For this review, take the finished solid that the model builds, in its own axes (mm). Give positions to 0.01 mm unless a question says otherwise; leave off trailing zeros. Write each loop counter-clockwise with the first axis right and the second up, starting at its lowest first coordinate (ties: lowest second). Pieces come first, ordered by that corner, then holes. Notation, with made-up numbers: M 29.25,64 L 69.25,64 A9 cw 69.25,77 Z; hole C -37,43.5 d3. An arc over 180 degrees is marked long. Answer as a JSON object with one key per item and string values. Group by question number.
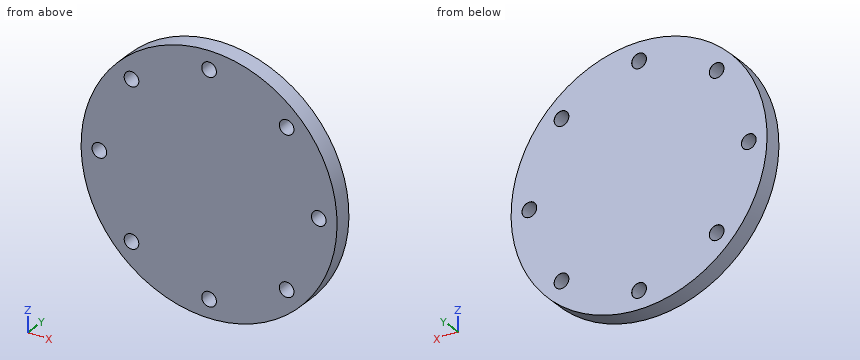
```python
from build123d import *

# Parameters (mm, degrees)
SKETCH_1_W                   = 70
SKETCH_1_H                   = 10
HOLE_WIZARD_M8_1_D           = 8
HOLE_WIZARD_M8_1_CSINK_D     = 8.05
HOLE_WIZARD_M8_1_CSINK_ANGLE = 100
PATTERN_CIRCULAR_2_COUNT     = 8


with BuildPart() as part:
    # Sketch 1 → Revolve 1 (revolve)
    with BuildSketch(Plane.XY, mode=Mode.PRIVATE) as revolve_1_sk:
        with Locations((-35, 5)):
            Rectangle(SKETCH_1_W, SKETCH_1_H)
    revolve(revolve_1_sk.sketch.rotate(Axis((0, 76.619497233, 0), (0, -1, 0)), 270), axis=Axis((0, 76.619497233, 0), (0, -1, 0)))

    # Hole Wizard M8 _1 (through all)
    with Locations(Plane(origin=(0, 10, 0), x_dir=(1, 0, 0), z_dir=(0, 1, 0))):
        with Locations((-60, 0)):
            hole_wizard_m8_1 = CounterSinkHole(HOLE_WIZARD_M8_1_D / 2, HOLE_WIZARD_M8_1_CSINK_D / 2, counter_sink_angle=HOLE_WIZARD_M8_1_CSINK_ANGLE)

    # Pattern Circular 2: Hole Wizard M8 _1 ×8 about axis
    pattern_circular_2_axis = Axis((0, 0, 0), (0, 1, 0))
    for i in range(1, PATTERN_CIRCULAR_2_COUNT):
        add(hole_wizard_m8_1.rotate(pattern_circular_2_axis, i * 360 / PATTERN_CIRCULAR_2_COUNT), mode=Mode.SUBTRACT)


solid = part.part
```
Item 1: Insertion check: P1, Ø6.5, axis at x = 0, z = -60, coming from the +Y side; P2, Ø6, axis at x = 14.5, y = 6.5, coming from the -Z side; P3, Ø1, axis at y = 7, z = -3.5, coming from the +X side; P4, Ø1, axis at y = 6.5, z = -6.5, coming from the +X side. Each pin has a flat end and moves straight along its axis. Give the tip position at first contact, or say it passes through.
Item 2: Consider section B-B (x = 0). Give the boundary of the cut face in (y, z) (3 decimals).
Item 3: Consider section C-C (y = 4.5). State how many separate pieces and enclosed holes the cut face has, plus the area to 3 significant figures.
Item 4: Consider section D-D (z = -60). Give the boundary of the cut face in (x, y) (3 decimals).
Item 5: To check wall thickness, follow probe 1 along X at (y, z) = (1.25, 42); probe 2 along Z at (x, y) = (-1.5, 1.25); probe 3 along Z at (x, y) = (-3, 5.25). State the ranges of each line that lie inside material, in increasing order.
Item 6: Consider section A-A (z = 0). Give the boundary of the cut face in (x, y) (3 decimals), plus the area to 3 significant figures.
Result set:
{
 "1": {"P1": "passes through", "P2": "stops at z = -69.05", "P3": "stops at x = 69.94", "P4": "stops at x = 69.74"},
 "2": {"outline": "M 0,-70 L 10,-70 L 10,-64.025 L 9.979,-64 L 0,-64 Z; M 0,-56 L 9.979,-56 L 10,-55.975 L 10,55.975 L 9.979,56 L 0,56 Z; M 0,64 L 9.979,64 L 10,64.025 L 10,70 L 0,70 Z"},
 "3": {"separate pieces": "1", "enclosed holes": "8", "area": "15,000 mm^2"},
 "4": {"outline": "M -36.056,0 L -4,0 L -4,9.979 L -4.025,10 L -36.056,10 Z; M 4,0 L 36.056,0 L 36.056,10 L 4.025,10 L 4,9.979 Z"},
 "5": {"probe 1": "x = -56 to -46.4, -38.45 to 38.45, 46.4 to 56", "probe 2": "z = -69.98 to -63.71, -56.29 to 56.29, 63.71 to 69.98", "probe 3": "z = -69.94 to -62.65, -57.35 to 57.35, 62.65 to 69.94"},
 "6": {"outline": "M -70,0 L -64,0 L -64,9.979 L -64.025,10 L -70,10 Z; M -56,0 L 56,0 L 56,9.979 L 55.975,10 L -55.975,10 L -56,9.979 Z; M 64,0 L 70,0 L 70,10 L 64.025,10 L 64,9.979 Z", "area": "1,240 mm^2"}
}
